Could you check a few things on this model? Use its own coordinates, in mm. A direction names the side the tool comes from. Coordinates: 2 decimals unless noted, no trailing zeros. Order: outer loops, then holes, each group sorted by start corner. A loop starts at its lowest first (then second) coordinate and runs counter-clockwise, first axis right, second up. Notation, with made-up numbers: (68.5, 15.25) - (96.5, 15.25) arc R28 cw to (96.5, 50.25) - close; hole circle Ø3 at (-26.5, 68.25). An arc over 180 degrees is marked (long way). Answer as a JSON object with one key per item and string values. Group by question number.
(1) Imagine slicing it at A-A, the plane x = 0. Write out the boundary of the cut face in (y, z).
(2) Imagine slicing it at B-B, the plane x = 13. Write out the boundary of the cut face in (y, z).
(3) Please list where these lines run through material, in increasing order: probe 1 along X at (y, z) = (-18.9, 0.25); probe 2 along Y at (x, z) = (13, 1.8); probe 3 along X at (y, z) = (0, 1.55).
(4) We'd pull the mould along Y, two halves only. Please class faces 1 (the flat face through (-18.33, -17.95, 1.21)), 2 (the flat face through (0, -22.9, 1)), 3 (the cylindrical face through (16.4, 3.43, 1.01)): pulls with the +Y half, pulls with the -Y half, needs draft (parallel to the pull), parting line crosses it, or undercut.
(5) Imagine slicing it at D-D, the plane x = 20. Write out the boundary of the cut face in (y, z), and give its area (3 significant figures).
(6) Imagine slicing it at C-C, the plane y = -10.5. Write out the boundary of the cut face in (x, z), and give its area (3 significant figures).
(7) Will these pins go through, and if not, where does the flat tip stop? P1, Ø1.1, axis at y = 3.5, z = 1, coming from the +X side; P2, Ø0.6, axis at y = 0.5, z = 0.5, coming from the -X side; P3, Ø1.2, axis at x = 19.5, y = -18.5, coming from the +Z side.
(8) Which directions (+Z, -Z, +X, -X, +Y, -Y) give clear straight access to the entire face, cutting with the end or side of a thin tool? Please do faces 4 (the flat face through (1.67, 2.05, 1.21)), 5 (the flat face through (11.33, -0.95, 0.59)), 6 (the flat face through (0, -0.82, 1)).
from build123d import *

# Parameters (mm, degrees)
F2_DEPTH = 2
F3_R     = 1.1
F4_DEPTH = 2
F6_DEPTH = 1.2
F7_W     = 2.2170250337
F7_H     = 0.98
F8_DEPTH = 1.6
F9_R     = 2
F10_R    = 5
F11_R    = 3


with BuildPart() as f2:
    # F1 (on Top) → F2 (new body)
    with BuildSketch(Plane.XY):
        Polygon((0, 4), (-3, 4), (-13, 4), (-17, 4), (-17, -3.6), (-24, -16.9), (-24, -22.9), (0, -22.9), (24, -22.9), (24, -16.9), (17, -3.6), (17, 4), (13, 4), (3, 4), align=None)
    extrude(amount=F2_DEPTH)

    # F3 (on face) → F4 (cut, through all)
    with BuildSketch(Plane(origin=(0, 0, 0), x_dir=(1, 0, 0), z_dir=(0, 0, -1))):
        with Locations((20, 18.9)):
            Circle(F3_R)
        with Locations((13, 0)):
            Circle(F3_R)
        with Locations((0, -1.1)):
            Circle(F3_R)
        with Locations((-13, 0)):
            Circle(F3_R)
        with Locations((-20, 18.9)):
            Circle(F3_R)
    extrude(amount=-F4_DEPTH, mode=Mode.SUBTRACT)

    # F5 (on Top) → F6 (cut)
    with BuildSketch(Plane.XY):
        Polygon((10.7829749663, 0), (11.8914874832, -1.92), (14.1085125168, -1.92), (15.2170250337, 0), (14.1085125168, 1.92), (11.8914874832, 1.92), align=None)
        Polygon((-14.1085125168, -1.92), (-11.8914874832, -1.92), (-10.7829749663, 0), (-11.8914874832, 1.92), (-14.1085125168, 1.92), (-15.2170250337, 0), align=None)
    extrude(amount=F6_DEPTH, mode=Mode.SUBTRACT)

    # F7 (on face) → F8 (cut)
    with BuildSketch(Plane.XY.offset(2)):
        Polygon((-17.7829749663, -18.9), (-18.8914874832, -16.98), (-21.1085125168, -16.98), (-22.2170250337, -18.9), (-21.1085125168, -20.82), (-18.8914874832, -20.82), align=None)
        with Locations((0, 3.51)):
            Rectangle(F7_W, F7_H)
        Polygon((1.1085125168, 3.02), (-1.1085125168, 3.02), (-2.2170250337, 1.1), (-1.1085125168, -0.82), (1.1085125168, -0.82), (2.2170250337, 1.1), align=None)
        Polygon((18.8914874832, -16.98), (17.7829749663, -18.9), (18.8914874832, -20.82), (21.1085125168, -20.82), (22.2170250337, -18.9), (21.1085125168, -16.98), align=None)
    extrude(amount=-F8_DEPTH, mode=Mode.SUBTRACT)

    # F9
    f9_edges = [f2.edges().sort_by_distance(p)[0] for p in [
        (-17, 4, 1),
        (17, 4, 1),
    ]]
    fillet(f9_edges, radius=F9_R)

    # F10
    f10_edges = [f2.edges().sort_by_distance(p)[0] for p in [
        (24, -16.9, 1),
        (-24, -16.9, 1),
    ]]
    fillet(f10_edges, radius=F10_R)

    # F11
    f11_edges = [f2.edges().sort_by_distance(p)[0] for p in [
        (24, -22.9, 1),
        (-24, -22.9, 1),
    ]]
    fillet(f11_edges, radius=F11_R)


solid = f2.part
Result set:
{
 "1": {"outline": "(-22.9, 0) - (0, 0) - (0, 0.4) - (-0.82, 0.4) - (-0.82, 2) - (-22.9, 2) - close; (2.2, 0) - (4, 0) - (4, 0.4) - (2.2, 0.4) - close"},
 "2": {"outline": "(-22.9, 0) - (-1.92, 0) - (-1.92, 1.2) - (-1.1, 1.2) - (-1.1, 2) - (-22.9, 2) - close; (1.1, 1.2) - (1.92, 1.2) - (1.92, 0) - (4, 0) - (4, 2) - (1.1, 2) - close"},
 "3": {"probe 1": "x = -24 to -21.1, -18.9 to 18.9, 21.1 to 24", "probe 2": "y = -22.9 to -1.1, 1.1 to 4", "probe 3": "x = -17 to -14.1, -11.9 to -1.58, 1.58 to 11.9, 14.1 to 17"},
 "4": {"face 1": "undercut", "face 2": "pulls with the -Y half", "face 3": "pulls with the +Y half"},
 "5": {"outline": "(-22.9, 0) - (-20, 0) - (-20, 0.4) - (-20.82, 0.4) - (-20.82, 2) - (-22.9, 2) - close; (-17.8, 0) - (-9.3, 0) - (-9.3, 2) - (-16.98, 2) - (-16.98, 0.4) - (-17.8, 0.4) - close", "area": "20.2 mm^2"},
 "6": {"outline": "(-20.63, 0) - (20.63, 0) - (20.63, 2) - (-20.63, 2) - close", "area": "82.5 mm^2"},
 "7": {"P1": "stops at x = 16.76", "P2": "stops at x = -17", "P3": "stops at z = 0.4"},
 "8": {"face 4": "+Z", "face 5": "-Z", "face 6": "+Z, +Y"}
}
